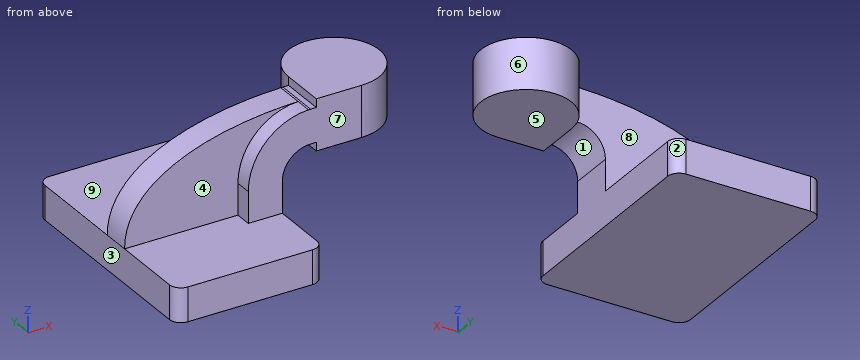
```python
from build123d import *

# Parameters (mm, degrees)
F1_DEPTH = 63.5
F2_DEPTH = 25.4
F3_DEPTH = 15.875
F4_R     = 6.35
F0_W     = 25.4
F0_H     = 28.575


with BuildPart() as f1:
    # F0 (on Front) → F1 (new body, symmetric)
    with BuildSketch(Plane.XZ):
        Polygon((22.225, 9.525), (-41.275, 9.525), (-41.275, -9.525), (41.275, -9.525), (41.275, 9.525), align=None)
    extrude(amount=F1_DEPTH, both=True)

    # F0 (on Front) → F2 (join)
    with BuildSketch(Plane.XZ):
        with BuildLine():
            Line((22.225, 27.0002), (22.225, 9.525))
            Line((22.225, 9.525), (41.275, 9.525))
            Line((41.275, 9.525), (41.275, 27.0002))
            ThreePointArc((41.275, 27.0002), (45.92468, 38.22552), (57.15, 42.8752))
            Line((57.15, 42.8752), (60.325, 42.8752))
            Line((60.325, 42.8752), (60.325, 61.9252))
            Line((60.325, 61.9252), (57.15, 61.9252))
            add(Edge.make_bspline(
                [(55.959567, 61.904906), (56.355854, 61.91256), (56.75267, 61.919325), (57.15, 61.9252)],
                knots=[110.684323, 110.684323, 110.684323, 110.684323, 111.504536, 111.504536, 111.504536, 111.504536], degree=3))
            ThreePointArc((55.959567, 61.904906), (32.036941, 51.271374), (22.225, 27.0002))
        make_face()
        Polygon((60.325, 66.675), (60.325, 61.9252), (60.325, 42.8752), (60.325, 38.1), (85.725, 38.1), (85.725, 66.675), align=None)
    extrude(amount=F2_DEPTH)

    # F0 (on Front) → F3 (join)
    with BuildSketch(Plane.XZ):
        with BuildLine():
            add(Edge.make_bspline(
                [(-41.275, 9.525), (-41.377201, 43.632958), (2.482248, 60.871958), (55.959567, 61.904906)],
                knots=[0, 0, 0, 0, 110.684323, 110.684323, 110.684323, 110.684323], degree=3))
            Line((-41.275, 9.525), (22.225, 9.525))
            Line((22.225, 9.525), (22.225, 27.0002))
            ThreePointArc((22.225, 27.0002), (32.036941, 51.271374), (55.959567, 61.904906))
        make_face()
    extrude(amount=F3_DEPTH)

    # F4
    f4_edges = [f1.edges().sort_by_distance(p)[0] for p in [
        (-41.275, -63.5, 0),
        (41.275, -63.5, 0),
        (41.275, 63.5, 0),
        (-41.275, 63.5, 0),
    ]]
    fillet(f4_edges, radius=F4_R)

    # F0 (on Front) → F5 (revolve)
    with BuildSketch(Plane.XZ):
        with Locations((98.425, 52.3875)):
            Rectangle(F0_W, F0_H)
    revolve(axis=Axis((85.725, 0, 52.3875), (0, 0, -1)))


solid = f1.part
```
The listing builds one solid part. Answer for the finished solid, in the listing's coordinates (mm). Face numbers are marked on the shaded views. A direction names the side the tool comes from. Give positions to 0.01 mm unless a question says otherwise; leave off trailing zeros. Order: outer loops, then holes, each group sorted by start corner. A loop starts at its lowest first (then second) coordinate and runs counter-clockwise, first axis right, second up. Notation, with made-up numbers: (27.25, -7) - (39.25, -7) arc R10 ccw to (39.25, 5) - close; hole circle Ø11 at (43, 48.5). An arc over 180 degrees is marked (long way). Use one line per item in the form item = value. Start each with the question number.
(1) The mould has two halves that part along X. Classify the marked faces 1, 2, 3 and 4: released by +X, released by -X, zero draft, split by the parting line, or undercut.
(2) A cutting plane is placed at B-B, the plane y = -42. Write down the section's boundary in (x, z) (3 decimals).
(3) Flat-ended cylindrical pins translate along their axes: pin 1 Ø5.5 at (y, z) = (-11.5, 40.5) entering from -X; pin 2 Ø15.5 at (x, z) = (11.5, 46.5) entering from +Y; pin 3 Ø1.5 at (x, z) = (16.5, 57.5) entering from -Y (3 decimals). Find the tip coordinate at first contact, or state that the pin passes through.
(4) A cutting plane is placed at A-A, the plane y = 22.5. Write down the section's boundary in (x, z) (3 decimals).
(5) For the marked faces 5, 6, 7, 8 and 9, determine the directions among +Z, -Z, +X, -X, +Y, -Y from which every point of the face is accessible in a straight line to the end or side of a thin tool.
(6) Consider line 1 (Z direction, x = 37.5, y = 8) (3 decimals); line 2 (Y direction, x = -15.5, z = 13) (3 decimals); line 3 (Y direction, x = 35, z = 22). Determine where each line is inside the solid, lowest interval first. Write a range as from..to.
Ans:
q1.face_1 = undercut
q1.face_2 = released by +X
q1.face_3 = released by -X
q1.face_4 = zero draft
q2.outline = (-41.275, -9.525) - (41.275, -9.525) - (41.275, 9.525) - (-41.275, 9.525) - close
q3.pin_1 = -28.31
q3.pin_2 = 0
q3.pin_3 = -15.875
q4.outline = (-41.275, -9.525) - (41.275, -9.525) - (41.275, 9.525) - (-41.275, 9.525) - close; (73.939, 38.1) - (97.511, 38.1) - (97.511, 66.675) - (73.939, 66.675) - close
q5.face_5 = -Z, +X, +Y, -Y
q5.face_6 = +Z, -Z
q5.face_7 = +Z, +X, -X, -Y
q5.face_8 = +Z, -X, +Y
q5.face_9 = +Z, +X, -X, +Y
q6.line_1 = -9.525..9.525
q6.line_2 = -15.875..0
q6.line_3 = -25.4..0
